Can you work these out from the drawing? Everything is in mm from the part's minimum corner. A direction names the side the tool comes from. Coordinates: 2 decimals unless noted, no trailing zeros. Order: outer loops, then holes, each group sorted by start corner. A loop starts at its lowest first (then second) coordinate and runs counter-clockwise, first axis right, second up. Notation, with made-up numbers: M -27,-24 L -23,-24 A28 ccw -23,10 Z; hole C 3,23.25 d1. An arc over 180 degrees is marked long. Answer as CSV lines item,"result". Start each with the question number.
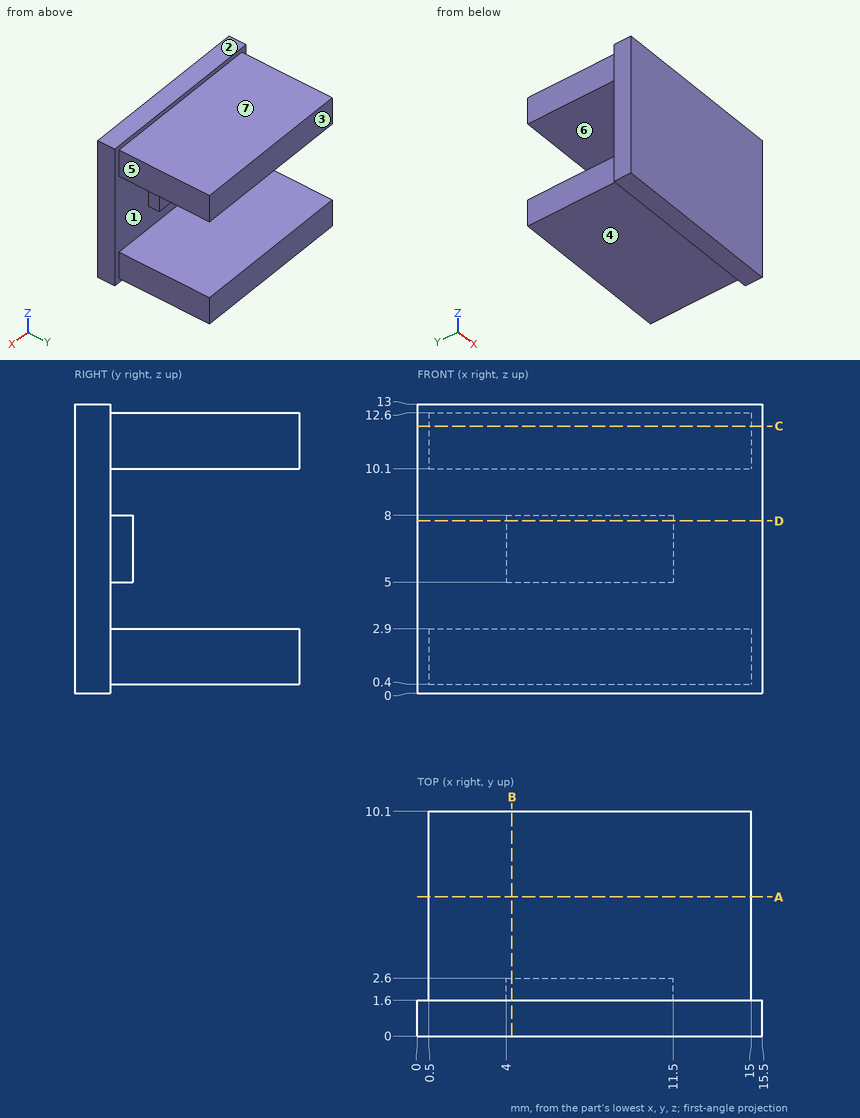
1) Suppose I cut it at C-C on z = 12. Please give me the cut outline in (x, y), plus the area to 3 significant figures.
2) If we mould it in two halves opening along Z, with no side actions, what happens to the marked faces 1, 2 and 3? For each: released by +Z, released by -Z, zero draft, split by the parting line, or undercut.
3) Suppose I cut it at D-D on z = 7.75. Please give me the cut outline in (x, y).
4) Which directions (+Z, -Z, +X, -X, +Y, -Y) give clear straight access to the entire face, cutting with the end or side of a thin tool? Please do the marked faces 4, 5, 6 and 7.
5) Will these pins go through, and if not, where does the flat tip stop? pin 1 Ø2 at (y, z) = (7, 1.5) entering from +X; pin 2 Ø0.5 at (x, y) = (9, 2) entering from -Z; pin 3 Ø2 at (y, z) = (4.5, 2) entering from -X.
6) Suppose I cut it at A-A on y = 6.25. Please give me the cut outline in (x, z).
7) Suppose I cut it at B-B on x = 4.25. Please give me the cut outline in (y, z), plus the area to 3 significant figures.
8) I need wall thicknesses on line 1 (Z direction, x = 5.5, y = 2); line 2 (Z direction, x = 8.5, y = 9); line 3 (Y direction, x = 13.25, z = 9.5). Which ranges of each line are inside material? Lowest first, please. Write a range as [from, to].
Output:
1,outline,"M 0,0 L 15.5,0 L 15.5,1.6 L 15,1.6 L 15,10.1 L 0.5,10.1 L 0.5,1.6 L 0,1.6 Z"
1,area,"148 mm²"
2,face 1,"undercut"
2,face 2,"released by +Z"
2,face 3,"zero draft"
3,outline,"M 0,0 L 15.5,0 L 15.5,1.6 L 11.5,1.6 L 11.5,2.6 L 4,2.6 L 4,1.6 L 0,1.6 Z"
4,face 4,"-Z, +X, -X, +Y"
4,face 5,"+Z, -Z, +X, +Y"
4,face 6,"+X, -X, +Y"
4,face 7,"+Z, +X, -X, +Y"
5,pin 1,"x = 15"
5,pin 2,"z = 0.4"
5,pin 3,"x = 0.5"
6,outline,"M 0.5,0.4 L 15,0.4 L 15,2.9 L 0.5,2.9 Z; M 0.5,10.1 L 15,10.1 L 15,12.6 L 0.5,12.6 Z"
7,outline,"M 0,0 L 1.6,0 L 1.6,0.4 L 10.1,0.4 L 10.1,2.9 L 1.6,2.9 L 1.6,5 L 2.6,5 L 2.6,8 L 1.6,8 L 1.6,10.1 L 10.1,10.1 L 10.1,12.6 L 1.6,12.6 L 1.6,13 L 0,13 Z"
7,area,"66.3 mm²"
8,line 1,"[0.4, 2.9], [5, 8], [10.1, 12.6]"
8,line 2,"[0.4, 2.9], [10.1, 12.6]"
8,line 3,"[0, 1.6]"
